Verification items for the finished model (mm, model axes). Face numbers are marked on the shaded views. Give positions to 0.01 mm unless a question says otherwise; leave off trailing zeros. Loops run counter-clockwise (first coordinate to the right, second up) from the corner with the lowest first, then second, coordinate; pieces in that order, holes last. Notation, with made-up numbers: (39, 68) -> (46, 68) arc R29 ccw to (46, 95) -> close; hole circle Ø6 at (14, 79). An arc over 180 degrees is marked (long way). Use one line per item in the form item = value. Start each with the question number.
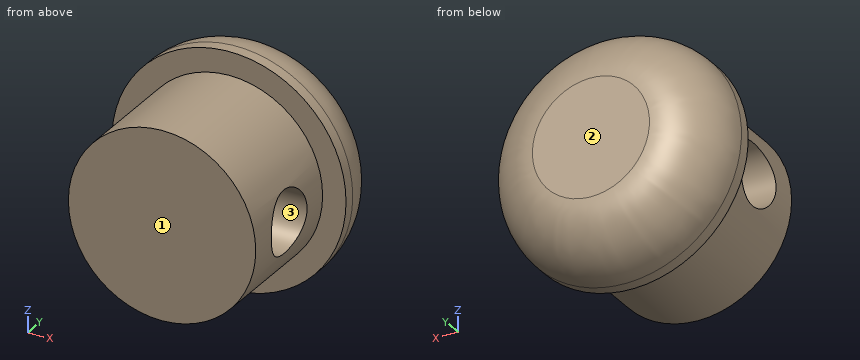
Autodesk Inventor part; units mm, degrees
ref_plane "Work Plane1" through (5.08, 0, 0) normal (1, 0, 0) x (0, 1, 0)
ref_plane "XZ Plane" through (0, 0, 0) normal (0, 1, 0) x (-1, 0, 0)
ref_plane "XY Plane" through (0, 0, 0) normal (0, 0, 1) x (1, 0, 0)
sketch "Sketch1" plane through (0, 0, 0) normal (0, 1, 0) x (-1, 0, 0)
  circle A0 centre (0, 0) radius 5.08
  dimension "d0" = 10.16
extrude "Extrusion1" add sketch "Sketch1" along normal blind 6.35
sketch "Sketch2" plane through (0, 6.35, 0) normal (0, 1, 0) x (1, 0, 0)
  circle A0 centre (0, 0) radius 6.35
  dimension "d3" = 12.7
extrude "Extrusion2" add sketch "Sketch2" along normal blind 3.81
fillet "Fillet1" radius 3.175 1 edges at (-6.35, 10.16, 0)
ref_plane "Work Plane1" through (5.08, 0, 0) normal (1, 0, 0) x (0, 1, 0)
sketch "Sketch3" plane through (5.08, 0, 0) normal (1, 0, 0) x (0, 1, 0)
  circle A0 centre (3.175, 0) radius 0.726
  point P0 (0, 0)
  dimension "d8" = 3.175
hole "Hole1" at (5.08, 3.175, 0) direction (-1, 0, 0) diameter 3.4 depth 25.4 tip angle 118
properties part number "Brass Endweight" material "Brass, Soft Yellow"
Item 1: Gauge pin test, flat ends, axial feed: pin 1 Ø2 at (x, z) = (5, 1.5) entering from +Y; pin 2 Ø6 at (x, y) = (-0.5, 1.5) entering from +Z; pin 3 Ø1 at (x, y) = (-0.5, 9) entering from +Z. Record the tip position at first contact, or that the pin passes through.
Item 2: Sectioned sample at A-A, the plane y = 2. Enter the section's corners in (x, z).
Item 3: Material ranges on line 1 (Y direction, x = 2.5, z = 0) (3 decimals); line 2 (Y direction, x = 2.25, z = 1.25); line 3 (Z direction, x = 3.25, y = 2.75), recorded low to high.
Item 4: Draft check along Y on the marked faces 1, 2 and 3. Enter one of: +Y half, -Y half, draft (parallel to the pull), parting line (faces both ways), or undercut.
Outcome:
q1.pin_1 = 9.98
q1.pin_2 = 5.08
q1.pin_3 = 5.95
q2.outline = (-4.93, -1.23) arc R5.08 ccw to (4.93, -1.23) -> close; (-4.93, 1.23) -> (4.93, 1.23) arc R5.08 ccw to start
q3.line_1 = 0 to 1.475, 4.875 to 10.16
q3.line_2 = 0 to 2.02, 4.33 to 10.16
q3.line_3 = -3.9 to -1.65, 1.65 to 3.9
q4.face_1 = -Y half
q4.face_2 = +Y half
q4.face_3 = undercut
